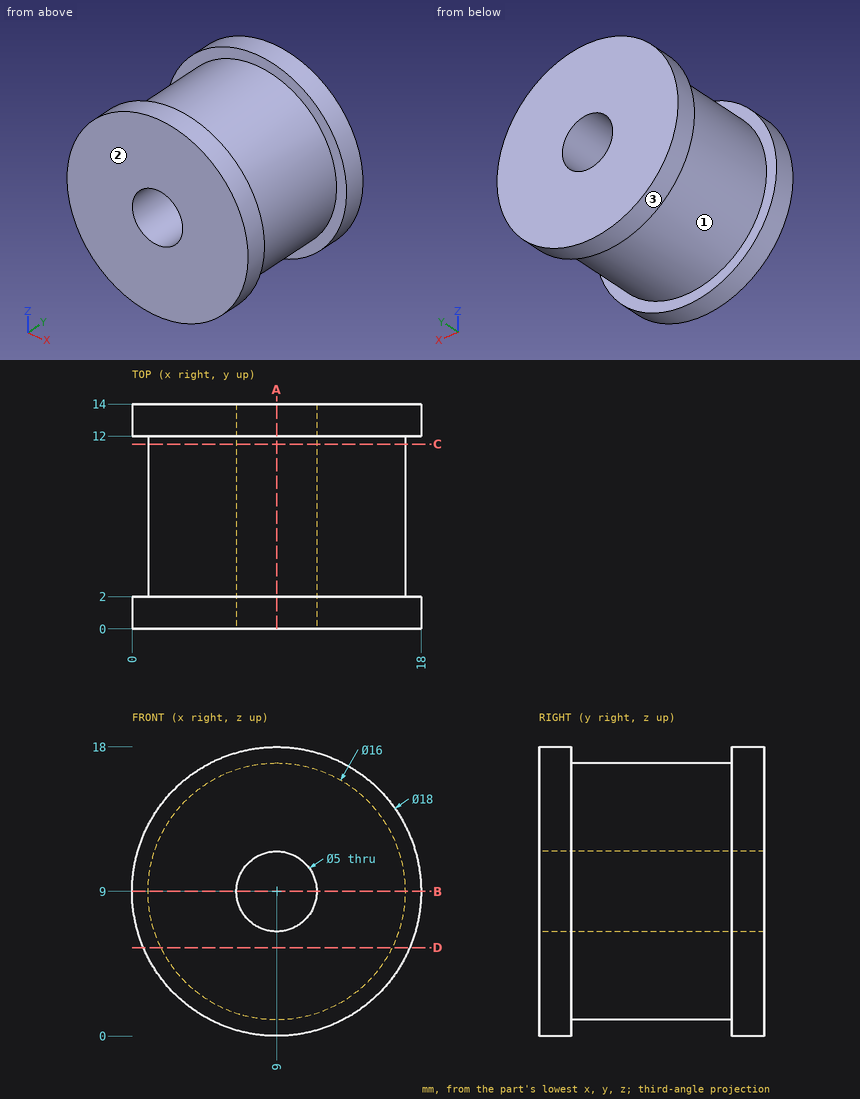
Print and shaded views of the part. All mm, measured from the part's lowest x, y and z. Round coordinates to 2 decimals unless told otherwise and drop trailing zeros. Order: outer loops, then holes, each group sorted by start corner. A loop starts at its lowest first (then second) coordinate and runs counter-clockwise, first axis right, second up. Notation, with made-up numbers: (-20.75, 66.5) - (1.25, 66.5) arc R18 cw to (1.25, 92.5) - close; hole circle Ø5 at (-34, 89). An arc over 180 degrees is marked (long way). Use a Markdown table: item, result.
1) Pull direction Y, two halves, no side cores. Call the marked faces 1, 2 and 3: pulls with the +Y half, pulls with the -Y half, needs draft (parallel to the pull), parting line crosses it, or undercut.
Recorded:
| item | result |
|---|---|
| face 1 | undercut |
| face 2 | pulls with the -Y half |
| face 3 | needs draft |
2) Saw through at C-C on y = 11.5. Write the cut outline in (x, z), and give its area (3 significant figures).
Recorded:
| item | result |
|---|---|
| outline | circle Ø16 at (9, 9); hole circle Ø5 at (9, 9) |
| area | 181 mm² |
3) Saw through at D-D on z = 5.5. Write the cut outline in (x, y).
Recorded:
| item | result |
|---|---|
| outline | (0.71, 0) - (17.29, 0) - (17.29, 2) - (16.19, 2) - (16.19, 12) - (17.29, 12) - (17.29, 14) - (0.71, 14) - (0.71, 12) - (1.81, 12) - (1.81, 2) - (0.71, 2) - close |
4) Saw through at B-B on z = 9. Write the cut outline in (x, y), and give its area (3 significant figures).
Recorded:
| item | result |
|---|---|
| outline | (0, 0) - (6.5, 0) - (6.5, 14) - (0, 14) - (0, 12) - (1, 12) - (1, 2) - (0, 2) - close; (11.5, 0) - (18, 0) - (18, 2) - (17, 2) - (17, 12) - (18, 12) - (18, 14) - (11.5, 14) - close |
| area | 162 mm² |
5) Saw through at A-A on x = 9. Write the cut outline in (y, z), and give its area (3 significant figures).
Recorded:
| item | result |
|---|---|
| outline | (0, 0) - (2, 0) - (2, 1) - (12, 1) - (12, 0) - (14, 0) - (14, 6.5) - (0, 6.5) - close; (0, 11.5) - (14, 11.5) - (14, 18) - (12, 18) - (12, 17) - (2, 17) - (2, 18) - (0, 18) - close |
| area | 162 mm² |
6) Flat gauge pins, fed straight in: pin 1 Ø5 at (y, z) = (8.5, 7.5) entering from -X; pin 2 Ø1.5 at (y, z) = (6, 8.5) entering from +X; pin 3 Ø6 at (y, z) = (11.5, 4.5) entering from -X. Where does each tip first touch, or does it go through?
Recorded:
| item | result |
|---|---|
| pin 1 | stops at x = 1 |
| pin 2 | stops at x = 17 |
| pin 3 | stops at x = 0.13 |
7) Wall check: L1, parallel to Y at x = 2.25, z = 3.5; L2, parallel to X at y = 8.5, z = 9; L3, parallel to Z at x = 7.25, y = 4.5. Give the ranges that are in metal, low to high.
Recorded:
| item | result |
|---|---|
| L1 | y = 0 to 2, 12 to 14 |
| L2 | x = 1 to 6.5, 11.5 to 17 |
| L3 | z = 1.19 to 7.21, 10.79 to 16.81 |
